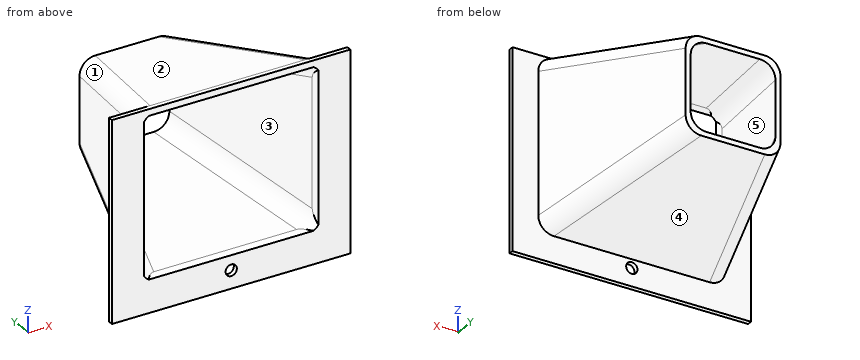
from build123d import *

# Parameters (mm, degrees)
SKETCH1_W           = 59
SKETCH1_H           = 59
BOSS_EXTRUDE1_DEPTH = 100
DRAFT1_ANGLE        = 13
DRAFT2_ANGLE        = 16
SHELL1_T            = -3
CUT_EXTRUDE3_REACH  = 126.734
SKETCH7_W           = 108.386808222
SKETCH7_H           = 97.630604432
SKETCH8_W           = 148.386808222
SKETCH8_H           = 137.630604432
SKETCH8_W_2         = 108.386808222
SKETCH8_H_2         = 97.630604432
BOSS_EXTRUDE7_DEPTH = 3
FILLET5_R           = 10
SKETCH9_R           = 3.5
CUT_EXTRUDE4_DEPTH  = 3
CUT_EXTRUDE5_REACH  = 146.393
SKETCH10_W          = 148.386808222
SKETCH10_H          = 16


with BuildPart() as part:
    # Sketch1 → Boss-Extrude1 (new body)
    with BuildSketch(Plane(origin=(0, 0, 0), x_dir=(1, 0, 0), z_dir=(0, 1, 0))):
        Rectangle(SKETCH1_W, SKETCH1_H)
    extrude(amount=-BOSS_EXTRUDE1_DEPTH)

    # Draft1
    draft1_faces = [part.faces().sort_by_distance(p)[0] for p in [
        (0, -50, 29.5),
        (0, -50, -29.5),
    ]]
    draft(draft1_faces, Plane.ZX, DRAFT1_ANGLE)

    # Draft2
    draft2_faces = [part.faces().sort_by_distance(p)[0] for p in [
        (-29.5, -54.687479947, 0),
        (29.5, -54.687479947, 0),
    ]]
    draft(draft2_faces, Plane.ZX, DRAFT2_ANGLE)

    # Shell1
    shell1_openings = [part.faces().sort_by_distance(p)[0] for p in [
        (0, 0, 0),
    ]]
    offset(amount=SHELL1_T, openings=shell1_openings, kind=Kind.INTERSECTION)

    # Sketch7 → Cut-Extrude3 (cut, up to next)
    with BuildSketch(Plane(origin=(0, -97, 0), x_dir=(1, 0, 0), z_dir=(0, 1, 0)), mode=Mode.PRIVATE) as cut_extrude3_sk1:
        Rectangle(SKETCH7_W, SKETCH7_H)
    cut_extrude3_tool1 = extrude(cut_extrude3_sk1.sketch, amount=-CUT_EXTRUDE3_REACH, mode=Mode.PRIVATE) & part.part
    add(cut_extrude3_tool1.solids().sort_by_distance((0, -97, 0))[0], mode=Mode.SUBTRACT)

    # Sketch8 → Boss-Extrude7 (add)
    with BuildSketch(Plane.XZ.offset(100)):
        Rectangle(SKETCH8_W, SKETCH8_H)
        Rectangle(SKETCH8_W_2, SKETCH8_H_2, mode=Mode.SUBTRACT)
    extrude(amount=BOSS_EXTRUDE7_DEPTH)

    # Fillet5
    # the kernel refuses this fillet: 10 mm, written as the material it adds along each edge
    with BuildSketch(Plane(origin=(60.515709798, -119.048500171, 53.905599567), x_dir=(0.05971785506372287, -0.20826091030442337, -0.9762485190901757), z_dir=(-0.26909056042227797, 0.9384303071178944, -0.2166537075017155))) as fillet5_piece_1_section:
        with BuildLine():
            CenterArc((FILLET5_R * 0.939803414436, FILLET5_R), FILLET5_R, 183.554900224, 86.445099776)
            Line((-FILLET5_R * 0.0582724297082, FILLET5_R * 0.937995086192), (0, 0))
            Line((0, 0), (FILLET5_R * 0.939803414436, 0))
        make_face()
    fillet5_piece_1 = extrude(amount=150.354266344, mode=Mode.PRIVATE)
    fillet5_piece_1 = split(fillet5_piece_1, bisect_by=Plane(origin=(38.566536387, -103, 35.845693728), z_dir=(0, 1, 0)), keep=Keep.TOP, mode=Mode.PRIVATE)
    fillet5_piece_1 = split(fillet5_piece_1, bisect_by=Plane(origin=(38.566536387, 0, 35.845693728), z_dir=(0, -1, 0)), keep=Keep.TOP, mode=Mode.PRIVATE)
    add(fillet5_piece_1)
    with BuildSketch(Plane(origin=(60.515709798, -119.048500171, -53.905599567), x_dir=(0.059717855063722874, -0.2082609103044234, 0.9762485190901756), z_dir=(-0.26909056042227797, 0.9384303071178944, 0.2166537075017155))) as fillet5_piece_2_section:
        with BuildLine():
            CenterArc((FILLET5_R * 0.939803414436, -FILLET5_R), FILLET5_R, 90, 86.445099776)
            Line((-FILLET5_R * 0.0582724297082, -FILLET5_R * 0.937995086192), (0, 0))
            Line((0, 0), (FILLET5_R * 0.939803414436, 0))
        make_face()
    fillet5_piece_2 = extrude(amount=150.354266344, mode=Mode.PRIVATE)
    fillet5_piece_2 = split(fillet5_piece_2, bisect_by=Plane(origin=(38.566536387, -103, -35.845693728), z_dir=(0, 1, 0)), keep=Keep.TOP, mode=Mode.PRIVATE)
    fillet5_piece_2 = split(fillet5_piece_2, bisect_by=Plane(origin=(38.566536387, 0, -35.845693728), z_dir=(0, -1, 0)), keep=Keep.TOP, mode=Mode.PRIVATE)
    add(fillet5_piece_2)
    with BuildSketch(Plane(origin=(-60.515709798, -119.048500171, -53.905599567), x_dir=(0.9631148790729092, -0.26219378679175015, -0.06053220528097297), z_dir=(0.26909056042227797, 0.9384303071178944, 0.2166537075017155))) as fillet5_piece_3_section:
        with BuildLine():
            CenterArc((FILLET5_R * 0.939803414436, -FILLET5_R), FILLET5_R, 90, 86.445099776)
            Line((-FILLET5_R * 0.0582724297082, -FILLET5_R * 0.937995086192), (0, 0))
            Line((0, 0), (FILLET5_R * 0.939803414436, 0))
        make_face()
    fillet5_piece_3 = extrude(amount=150.354266344, mode=Mode.PRIVATE)
    fillet5_piece_3 = split(fillet5_piece_3, bisect_by=Plane(origin=(-38.566536387, -103, -35.845693728), z_dir=(0, 1, 0)), keep=Keep.TOP, mode=Mode.PRIVATE)
    fillet5_piece_3 = split(fillet5_piece_3, bisect_by=Plane(origin=(-38.566536387, 0, -35.845693728), z_dir=(0, -1, 0)), keep=Keep.TOP, mode=Mode.PRIVATE)
    add(fillet5_piece_3)
    with BuildSketch(Plane(origin=(-20.056796005, 22.048500171, 21.330790325), x_dir=(-0.059717855063722264, -0.2082609103044235, -0.9762485190901756), z_dir=(-0.26909056042227797, -0.9384303071178944, 0.2166537075017155))) as fillet5_piece_4_section:
        with BuildLine():
            CenterArc((FILLET5_R * 0.939803414436, FILLET5_R), FILLET5_R, 183.554900224, 86.445099776)
            Line((-FILLET5_R * 0.0582724297082, FILLET5_R * 0.937995086192), (0, 0))
            Line((0, 0), (FILLET5_R * 0.939803414436, 0))
        make_face()
    fillet5_piece_4 = extrude(amount=150.354266344, mode=Mode.PRIVATE)
    fillet5_piece_4 = split(fillet5_piece_4, bisect_by=Plane(origin=(-38.566536387, -103, 35.845693728), z_dir=(0, 1, 0)), keep=Keep.TOP, mode=Mode.PRIVATE)
    fillet5_piece_4 = split(fillet5_piece_4, bisect_by=Plane(origin=(-38.566536387, 0, 35.845693728), z_dir=(0, -1, 0)), keep=Keep.TOP, mode=Mode.PRIVATE)
    add(fillet5_piece_4)
    # the kernel refuses this fillet: 10 mm, written as the material it takes off along each edge
    with BuildSketch(Plane(origin=(-23.177694313, 22.048500171, -24.409702648), x_dir=(-0.05971785506372238, -0.20826091030442354, 0.9762485190901757), z_dir=(-0.26909056042227797, -0.9384303071178944, -0.2166537075017155))) as fillet5_2_piece_1_section:
        with BuildLine():
            CenterArc((FILLET5_R * 0.939803414436, -FILLET5_R), FILLET5_R, 90, 86.445099776)
            Line((-FILLET5_R * 0.0582724297082, -FILLET5_R * 0.937995086192), (0, 0))
            Line((0, 0), (FILLET5_R * 0.939803414436, 0))
        make_face()
    fillet5_2_piece_1 = extrude(amount=153.551094044, mode=Mode.PRIVATE)
    fillet5_2_piece_1 = split(fillet5_2_piece_1, bisect_by=Plane(origin=(-41.676990214, -100, -38.91219309), z_dir=(0, 1, 0)), keep=Keep.TOP, mode=Mode.PRIVATE)
    add(fillet5_2_piece_1, mode=Mode.SUBTRACT)
    with BuildSketch(Plane(origin=(23.177694313, 22.048500171, -24.409702648), x_dir=(0.059717855063722375, -0.2082609103044235, 0.9762485190901756), z_dir=(0.26909056042227797, -0.9384303071178944, -0.2166537075017155))) as fillet5_2_piece_2_section:
        with BuildLine():
            CenterArc((FILLET5_R * 0.939803414436, FILLET5_R), FILLET5_R, 183.554900224, 86.445099776)
            Line((-FILLET5_R * 0.0582724297082, FILLET5_R * 0.937995086192), (0, 0))
            Line((0, 0), (FILLET5_R * 0.939803414436, 0))
        make_face()
    fillet5_2_piece_2 = extrude(amount=153.551094044, mode=Mode.PRIVATE)
    fillet5_2_piece_2 = split(fillet5_2_piece_2, bisect_by=Plane(origin=(41.676990214, -100, -38.91219309), z_dir=(0, 1, 0)), keep=Keep.TOP, mode=Mode.PRIVATE)
    add(fillet5_2_piece_2, mode=Mode.SUBTRACT)
    with BuildSketch(Plane(origin=(23.177694313, 22.048500171, 24.409702648), x_dir=(-0.9631148790729092, -0.26219378679175015, 0.06053220528097312), z_dir=(0.26909056042227797, -0.9384303071178944, 0.2166537075017155))) as fillet5_2_piece_3_section:
        with BuildLine():
            CenterArc((FILLET5_R * 0.939803414436, FILLET5_R), FILLET5_R, 183.554900224, 86.445099776)
            Line((-FILLET5_R * 0.0582724297082, FILLET5_R * 0.937995086192), (0, 0))
            Line((0, 0), (FILLET5_R * 0.939803414436, 0))
        make_face()
    fillet5_2_piece_3 = extrude(amount=153.551094044, mode=Mode.PRIVATE)
    fillet5_2_piece_3 = split(fillet5_2_piece_3, bisect_by=Plane(origin=(41.676990214, -100, 38.91219309), z_dir=(0, 1, 0)), keep=Keep.TOP, mode=Mode.PRIVATE)
    add(fillet5_2_piece_3, mode=Mode.SUBTRACT)
    with BuildSketch(Plane(origin=(-23.177694313, 22.048500171, 24.409702648), x_dir=(0.9631148790729092, -0.26219378679175015, 0.06053220528097312), z_dir=(-0.26909056042227797, -0.9384303071178944, 0.2166537075017155))) as fillet5_2_piece_4_section:
        with BuildLine():
            CenterArc((FILLET5_R * 0.939803414436, -FILLET5_R), FILLET5_R, 90, 86.445099776)
            Line((-FILLET5_R * 0.0582724297082, -FILLET5_R * 0.937995086192), (0, 0))
            Line((0, 0), (FILLET5_R * 0.939803414436, 0))
        make_face()
    fillet5_2_piece_4 = extrude(amount=153.551094044, mode=Mode.PRIVATE)
    fillet5_2_piece_4 = split(fillet5_2_piece_4, bisect_by=Plane(origin=(-41.676990214, -100, 38.91219309), z_dir=(0, 1, 0)), keep=Keep.TOP, mode=Mode.PRIVATE)
    add(fillet5_2_piece_4, mode=Mode.SUBTRACT)

    # Sketch9 → Cut-Extrude4 (cut)
    with BuildSketch(Plane(origin=(0, -100, 0), x_dir=(1, 0, 0), z_dir=(0, 1, 0))):
        with Locations(Location((0, 57.815302216, 0), (0, 0, 270))):
            Circle(SKETCH9_R)
    extrude(amount=-CUT_EXTRUDE4_DEPTH, mode=Mode.SUBTRACT)

    # Sketch10 → Cut-Extrude5 (cut, up to next)
    with BuildSketch(Plane.XZ.offset(103), mode=Mode.PRIVATE) as cut_extrude5_sk1:
        with Locations((0, 60.815302216)):
            Rectangle(SKETCH10_W, SKETCH10_H)
    cut_extrude5_tool1 = extrude(cut_extrude5_sk1.sketch, amount=-CUT_EXTRUDE5_REACH, mode=Mode.PRIVATE) & part.part
    add(cut_extrude5_tool1.solids().sort_by_distance((0, -103, 60.815302))[0], mode=Mode.SUBTRACT)


solid = part.part
Here's how the part is built. I have some questions about the finished solid (model axes, mm). Face numbers are marked on the shaded views. A direction names the side the tool comes from. Round coordinates to 2 decimals unless told otherwise and drop trailing zeros. Write each loop counter-clockwise with the first axis right and the second up, starting at its lowest first coordinate (ties: lowest second). Pieces come first, ordered by that corner, then holes.
1. Suppose I cut it at B-B (x = 61). List the corners of the cut face in (y, z) for me, and give its area (3 significant figures).
2. If we mould it in two halves opening along X, with no side actions, what happens to the marked faces 1, 2 and 3? For each: released by +X, released by -X, zero draft, split by the parting line, or undercut.
3. I need wall thicknesses on L1, parallel to X at y = -61.5, z = 14; L2, parallel to Z at x = 32, y = -92; L3, parallel to X at y = -39.5, z = 21.5. Which ranges of each line are inside material? Lowest first, please.
4. For the marked faces 4 and 5, which set-ups out of +Z, -Z, +X, -X, +Y, -Y let a thin tool reach every point of the face, with its end or its side?
5. Suppose I cut it at A-A (x = 0). List the corners of the cut face in (y, z) for me, and give its area (3 significant figures).
6. Will these pins go through, and if not, where does the flat tip stop? pin 1 Ø1.8 at (x, y) = (-5, -98.5) entering from +Z; pin 2 Ø4 at (y, z) = (-25, -13) entering from -X; pin 3 Ø6 at (x, y) = (37, -88) entering from +Z.
Answer sheet:
1. outline: (-103, -68.82) - (-100, -68.82) - (-100, 52.82) - (-103, 52.82) - close
1. area: 365 mm2
2. face 1: released by -X
2. face 2: zero draft
2. face 3: undercut
3. L1: x = -47.13 to -44.01, 44.01 to 47.13
3. L2: z = -50.74 to -47.66, 47.66 to 50.74
3. L3: x = -40.83 to -37.71, 37.71 to 40.83
4. face 4: -Z, +X, -X, +Y
4. face 5: -Y
5. outline: (-103, -68.82) - (-100, -68.82) - (-100, -61.32) - (-103, -61.32) - close; (-103, -54.32) - (-100, -54.32) - (-100, -52.59) - (0, -29.5) - (0, -26.42) - (-97, -48.82) - (-103, -48.82) - close; (-103, 48.82) - (-97, 48.82) - (0, 26.42) - (0, 29.5) - (-100, 52.59) - (-100, 52.82) - (-103, 52.82) - close
5. area: 669 mm2
6. pin 1: stops at z = 52.45
6. pin 2: stops at x = -37.24
6. pin 3: stops at z = 50.51
